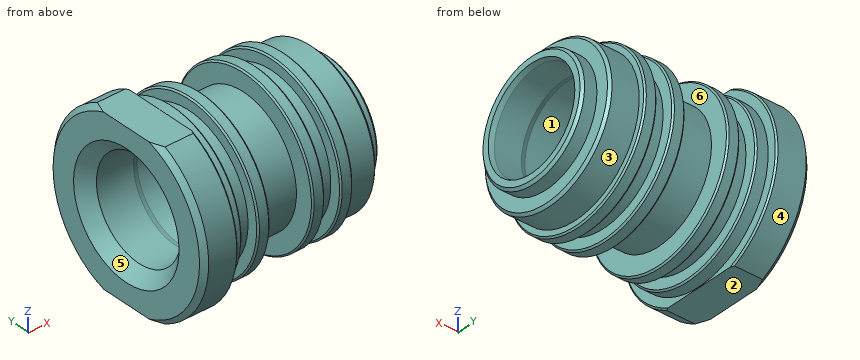
Autodesk Inventor part; units mm, degrees
ref_plane "YZ Plane" through (0, 0, 0) normal (1, 0, 0) x (0, 1, 0)
ref_plane "XZ Plane" through (0, 0, 0) normal (0, 1, 0) x (-1, 0, 0)
ref_plane "XY Plane" through (0, 0, 0) normal (0, 0, 1) x (1, 0, 0)
sketch "Náčrt1" plane through (0, 0, 0) normal (0, 0, 1) x (1, 0, 0)
  line L0 (0, 0) -> (20.108, 0)
  line L1 (0, 12.5) -> (0, 18.35)
  line L2 (0, 18.35) -> (7, 18.35)
  line L3 (7, 18.35) -> (7, 16.35)
  line L4 (7, 16.35) -> (9.5, 16.35)
  line L5 (9.5, 16.35) -> (9.5, 14)
  line L6 (9.5, 14) -> (12.7, 14)
  line L7 (12.7, 14) -> (12.7, 16.35)
  line L8 (12.7, 16.35) -> (15.2, 16.35)
  line L9 (15.2, 16.35) -> (15.2, 12.5)
  line L10 (15.2, 12.5) -> (23.8, 12.5)
  line L11 (23.8, 12.5) -> (23.8, 16.35)
  line L12 (23.8, 16.35) -> (26.3, 16.35)
  line L13 (26.3, 16.35) -> (26.3, 14)
  line L14 (26.3, 14) -> (29.5, 14)
  line L15 (29.5, 14) -> (29.5, 16.35)
  line L16 (29.5, 16.35) -> (32, 16.35)
  line L17 (32, 16.35) -> (32, 15)
  line L18 (32, 15) -> (38, 15)
  line L19 (38, 15) -> (38, 12)
  line L20 (38, 12) -> (41, 12)
  line L21 (41, 12) -> (41, 10.2679)
  line L22 (40, 10) -> (34.5, 10)
  line L23 (33.567, 10.25) -> (10.933, 10.25)
  line L24 (10, 10) -> (2.5, 10)
  line L25 (34.5, 10) -> (33.567, 10.25)
  line L26 (10, 10) -> (10.933, 10.25)
  line L27 (0, 12.5) -> (2.5, 10)
  line L28 (40, 10) -> (41, 10.2679)
  dimension "d0" = 41
  dimension "d1" = 36.7
  dimension "d2" = 24
  dimension "d3" = 30
  dimension "d4" = 3
  dimension "d5" = 9
  dimension "d6" = 32.7
  dimension "d7" = 25
  dimension "d9" = 20
  dimension "d10" = 20
  dimension "d11" = 20.5
  dimension "d15" = 34
  dimension "d16" = 2.5
  dimension "d17" = 2.5
  dimension "d18" = 2.5
  dimension "d19" = 2.5
  dimension "d20" = 3.2
  dimension "d21" = 3.2
  dimension "d23" = 28
  dimension "d24" = 15
  dimension "d25" = 15
  dimension "d50" = 25
  dimension "d51" = 10
  dimension "d52" = 2.5
  dimension "d53" = 45
  dimension "d54" = 6.5
  dimension "d55" = 15
  dimension "d56" = 1
revolve "Rotace1" add sketch "Náčrt1" angle 360 about axis through (0, 0, 0) along (1, 0, 0)
chamfer "Zkosení1" distance 1 angle 45 1 edges at (0, -18.35, 0)
chamfer "Zkosení2" distance 0.3 angle 45 1 edges at (7, -18.35, 0)
chamfer "Zkosení3" distance 0.5 angle 45 1 edges at (41, -12, 0)
chamfer "Zkosení4" distance 0.3 angle 45 7 edges at (32, -16.35, 0) (29.5, -16.35, 0) (26.3, -16.35, 0) (23.8, -16.35, 0) (15.2, -16.35, 0) (12.7, -16.35, 0) (9.5, -16.35, 0)
thread "Závit1"
chamfer "Zkosení5" distance 0.5 angle 45 1 edges at (38, -15, 0)
sketch "Náčrt2" plane through (0, 0, 0) normal (-1, 0, 0) x (0, 0, 1)
  line L0 (-20.0207, 8.0295) -> (-16.5, 8.0295)
  line L1 (-16.5, 8.0295) -> (-16.5, -8.0295)
  line L2 (-16.5, -8.0295) -> (-20.0207, -8.0295)
  line L3 (-20.0207, -8.0295) -> (-20.0207, 8.0295)
  line L4 (28.0067, 8.0295) -> (16.5, 8.0295)
  line L5 (16.5, 8.0295) -> (16.5, -8.0295)
  line L6 (16.5, -8.0295) -> (28.0067, -8.0295)
  line L7 (28.0067, -8.0295) -> (28.0067, 8.0295)
  circle A0 centre (0, 0) radius 18.35 construction
  line L8 (0, 0) -> (0, 5.8894) construction
  dimension "d46" = 33
extrude "Vysunutí1" cut sketch "Náčrt2" against normal through all
equation "\"d9\" = d10"
equation "\"Rozmer_A\" = d1"
equation "\"Rozmer_B\" = 0"
equation "\"Rozmer_C\" = 0"
equation "\"Rozmer_D\" = d0"
properties part number "NA-45-h-Crown-307" material "14 100"
Geometry check sheet. Reference: the model listing, model coordinates, mm. Face numbers are marked on the shaded views. A direction names the side the tool comes from. Round coordinates to 2 decimals unless told otherwise and drop trailing zeros. Order: outer loops, then holes, each group sorted by start corner. A loop starts at its lowest first (then second) coordinate and runs counter-clockwise, first axis right, second up. Notation, with made-up numbers: (72.5, 55.25) -> (90.5, 55.25) arc R17 ccw to (90.5, 67.25) -> close; hole circle Ø4 at (55, 8). An arc over 180 degrees is marked (long way). Use one line per item in the form item = value.
1. Cross-section at B-B, the plane x = 20. Enter the section's corners in (y, z).
Working result:
outline = circle Ø25 at (0, 0); hole circle Ø20.5 at (0, 0)
2. Scan lines: line 1 along X through (y, z) = (-11, -9); line 2 along X through (y, z) = (-13, -9); line 3 along X through (y, z) = (-11.5, 5.5). Record each from-to range of solid material in increasing order. Write a range as from..to.
Working result:
line_1 = 0..9.5, 12.7..15.2, 23.8..26.3, 29.5..38
line_2 = 0..9.5, 12.7..15.2, 23.8..26.3, 29.5..32
line_3 = 0..15.2, 23.8..38
3. Go/stop test with flat-tipped pins: pin 1 (8 mm diameter, centred on x = 32.5, y = -7.5, fed in from -Z); pin 2 (12 mm diameter, centred on x = 18, y = 7, fed in from +Z); pin 3 (2 mm diameter, centred on x = 31.5, y = -4.5, fed in from -Z); pin 4 (16 mm diameter, centred on y = -6.5, z = -3, fed in from -X). Record where each tip stops, or that it passes through.
Working result:
pin_1 = -15.95
pin_2 = 16.24
pin_3 = -15.97
pin_4 = 0
4. Cross-section at A-A, the plane x = 4. Enter the section's corners in (y, z).
Working result:
outline = (-8.03, -16.5) -> (8.03, -16.5) arc R18.35 ccw to (8.03, 16.5) -> (-8.03, 16.5) arc R18.35 ccw to start; hole circle Ø20 at (0, 0)
5. Mould release check, pull along X, two halves, no side actions. Record for the marked faces 4, 5 and 6: pulls with the +X half, pulls with the -X half, needs draft (parallel to the pull), parting line crosses it, or undercut.
Working result:
face_4 = needs draft
face_5 = pulls with the -X half
face_6 = undercut
6. Set-up check for the marked faces 1, 2 and 3: record each of +Z, -Z, +X, -X, +Y, -Y from which the full face is reachable in a straight line by a thin tool's end or side.
Working result:
face_1 = none
face_2 = -Z, +X, -X, +Y, -Y
face_3 = +X
7. Cross-section at C-C, the plane x = 27. Enter the section's corners in (y, z), plus the area to 3 significant figures.
Working result:
outline = circle Ø28 at (0, 0); hole circle Ø20.5 at (0, 0)
area = 286 mm^2
